Input: part model. Units: mm. Frame: model coordinates. A direction names the side the tool comes from. Round coordinates to 2 decimals unless told otherwise and drop trailing zeros. Write each loop counter-clockwise with the first axis right and the second up, starting at its lowest first coordinate (ties: lowest second). Pieces come first, ordered by that corner, then holes. Notation, with made-up numbers: (33, -10) -> (54, -10) arc R6 ccw to (54, -1) -> close; hole circle Ø8 at (-2.75, -28.75). An arc over 180 degrees is marked (long way). Write item = value, one per line.
Autodesk Inventor part; units mm, degrees
ref_plane "YZ Plane" through (0, 0, 0) normal (1, 0, 0) x (0, 1, 0)
ref_plane "XZ Plane" through (0, 0, 0) normal (0, 1, 0) x (-1, 0, 0)
ref_plane "XY Plane" through (0, 0, 0) normal (0, 0, 1) x (1, 0, 0)
sketch "Sketch1" plane through (0, 0, 0) normal (0, 0, 1) x (1, 0, 0)
  line L0 (0, 0) -> (0, 38.1)
  line L1 (0, 38.1) -> (12.7, 38.1)
  line L2 (12.7, 38.1) -> (12.7, 12.7)
  line L3 (12.7, 12.7) -> (4.445, 12.7)
  line L4 (4.445, 12.7) -> (4.445, 0)
  line L5 (4.445, 0) -> (0, 0)
  dimension "d0" = 38.1
  dimension "d1" = 12.7
  dimension "d2" = 25.4
  dimension "d3" = 8.255
revolve "Revolution1" add sketch "Sketch1" angle 360 about axis through (0, 0, 0) along (0, 1, 0)
sketch "Sketch2" plane through (0, 0, 0) normal (0, 0, 1) x (1, 0, 0)
  line L0 (-12.7, 38.1) -> (12.7, 38.1)
  line L1 (12.7, 38.1) -> (12.7, 12.7)
  line L2 (12.7, 12.7) -> (4.445, 12.7)
  line L3 (4.445, 12.7) -> (4.445, 0)
  line L4 (4.445, 0) -> (-4.445, 0)
  line L5 (-4.445, 0) -> (-4.445, 12.7)
  line L6 (-4.445, 12.7) -> (-12.7, 12.7)
  line L7 (-12.7, 12.7) -> (-12.7, 38.1)
  circle A0 centre (0, 25.4) radius 3.175
  point P0 (0, 0)
  dimension "d5" = 6.35
extrude "Extrusion1" cut sketch "Sketch2" along normal through all both and the other way through all contours A0
sketch "Sketch3" plane through (0, 0, 0) normal (1, 0, 0) x (0, 1, 0)
  line L0 (28.575, 12.7) -> (30.1625, 12.7)
  line L1 (30.1625, 12.7) -> (30.1625, 11.1125)
  line L2 (30.1625, 11.1125) -> (20.6375, 11.1125)
  line L3 (20.6375, 11.1125) -> (20.6375, 12.7)
  line L4 (20.6375, 12.7) -> (30.1625, 12.7)
  point P0 (0, 0)
  point P1 (38.1, 12.7)
  dimension "d9" = 1.5875
  dimension "d10" = 1.5875
  dimension "d11" = 9.525
extrude "Extrusion2" cut sketch "Sketch3" along normal through all both and the other way through all
sketch "Sketch4" plane through (0, 0, 0) normal (1, 0, 0) x (0, 1, 0)
  line L0 (38.1, -12.7) -> (12.7, -12.7)
  line L1 (38.1, -12.7) -> (28.575, -12.7)
  point P0 (0, 0)
  dimension "d14" = 9.525
properties part number "right angle rod holder"
1) Line query: L1, parallel to X at y = 25.4, z = -0.5 (3 decimals); L2, parallel to Y at x = 0, z = -0.5 (3 decimals); L3, parallel to Z at x = 0.5, y = 33. Output: solid intervals per line, ascending. Write a range as from..to.
Solutions:
L1 = -12.69..-3.175, 3.175..12.69
L2 = 0..22.225, 28.575..38.1
L3 = -12.69..12.69
2) Cut plane C-C (y = 25.4). Return the cut outline in (x, z) (1 decimal).
Solutions:
outline = (-6.1, 11.1) arc R12.7 ccw to (-3.2, -12.3) -> (-3.2, 11.1) -> close; (3.2, -12.3) arc R12.7 ccw to (6.1, 11.1) -> (3.2, 11.1) -> close
3) Cut plane A-A (x = -2.5). Return the cut outline in (y, z), and give its area (3 significant figures).
Solutions:
outline = (0, -3.68) -> (12.7, -3.68) -> (12.7, -12.45) -> (23.44, -12.45) -> (23.44, 11.11) -> (20.64, 11.11) -> (20.64, 12.45) -> (12.7, 12.45) -> (12.7, 3.68) -> (0, 3.68) -> close; (27.36, -12.45) -> (38.1, -12.45) -> (38.1, 12.45) -> (30.16, 12.45) -> (30.16, 11.11) -> (27.36, 11.11) -> close
area = 621 mm^2
4) Cut plane B-B (z = 0). Return the cut outline in (x, y) (3 decimals), and give its area (3 significant figures).
Solutions:
outline = (-12.7, 12.7) -> (-4.445, 12.7) -> (-4.445, 0) -> (4.445, 0) -> (4.445, 12.7) -> (12.7, 12.7) -> (12.7, 38.1) -> (-12.7, 38.1) -> close; hole circle Ø6.35 at (0, 25.4)
area = 726 mm^2
5) Draft query along Y for faces 4 (the face through (0, 38.1, 0)), 5 (the face through (0, 30.162, 12)), 6 (the face through (5, 12.7, 0)). Return one class per face: +Y half, -Y half, draft (parallel to the pull), parting line (faces both ways), or undercut.
Solutions:
face_4 = +Y half
face_5 = undercut
face_6 = -Y half
6) Cut plane D-D (x = 1). Return the cut outline in (y, z).
Solutions:
outline = (0, -4.33) -> (12.7, -4.33) -> (12.7, -12.66) -> (22.39, -12.66) -> (22.39, 11.11) -> (20.64, 11.11) -> (20.64, 12.66) -> (12.7, 12.66) -> (12.7, 4.33) -> (0, 4.33) -> close; (28.41, -12.66) -> (38.1, -12.66) -> (38.1, 12.66) -> (30.16, 12.66) -> (30.16, 11.11) -> (28.41, 11.11) -> close
7) First-contact query: P1, Ø8, axis at y = 34, z = 8, coming from the -X side; P2, Ø10, axis at y = 20, z = -0.5, coming from the +X side; P3, Ø1, axis at x = 7, y = 21, coming from the +Z side; P4, Ø3, axis at x = -2.5, y = 27, coming from the +Z side. Flat tips, straight axial feed; report the tip coordinate or a pass-through.
Solutions:
P1 = -12.05
P2 = 12.7
P3 = 10.91
P4 = 11.11
8) Access query for faces 1 (the face through (-0.96, 6.26, -4.34)), 2 (the face through (0, 0, 0)), 3 (the face through (0, 20.638, 12)). Directions: +Z, -Z, +X, -X, +Y, -Y. A direction counts if a zero-diameter tool reaches every point of the face in a straight line with its end or side. Return the directions, or none.
Solutions:
face_1 = -Y
face_2 = +Z, -Z, +X, -X, -Y
face_3 = +Z, +X, -X
